```python
from build123d import *

# Parameters (mm, degrees)
SKETCH1_R               = 2.5
EXTRUDE_1_DEPTH         = 50
HOLE_WIZARD_5_5_5_5_1_D = 5.5
HOLE_WIZARD_5_5_5_5_2_D = 5.5


with BuildPart() as part:
    # Sketch1 → 凸台-拉伸1 (new body)
    with BuildSketch(Plane.XY):
        with BuildLine():
            Line((-6, -15), (-3.25, -15))
            Line((-3.25, -15), (-3.25, -13))
            Line((-3.25, -13), (-5, -13))
            Line((-5, -13), (-5, -6))
            Line((-5, -6), (-3.25, -6))
            Line((-3.25, -6), (-3.25, -4))
            Line((-3.25, -4), (3.25, -4))
            Line((3.25, -4), (3.25, -6))
            Line((3.25, -6), (5, -6))
            Line((5, -6), (5, -13))
            Line((5, -13), (3.25, -13))
            Line((3.25, -13), (3.25, -15))
            Line((3.25, -15), (6, -15))
            ThreePointArc((6, -15), (7.060660172, -14.560660172), (7.5, -13.5))
            Line((7.5, -13.5), (7.5, 13.5))
            ThreePointArc((7.5, 13.5), (7.060660172, 14.560660172), (6, 15))
            Line((6, 15), (3.25, 15))
            Line((3.25, 15), (3.25, 13))
            Line((3.25, 13), (5, 13))
            Line((5, 13), (5, 6))
            Line((5, 6), (3.25, 6))
            Line((3.25, 6), (3.25, 4))
            Line((3.25, 4), (-3.25, 4))
            Line((-3.25, 4), (-3.25, 6))
            Line((-3.25, 6), (-5, 6))
            Line((-5, 6), (-5, 13))
            Line((-5, 13), (-3.25, 13))
            Line((-3.25, 13), (-3.25, 15))
            Line((-3.25, 15), (-6, 15))
            ThreePointArc((-6, 15), (-7.060660172, 14.560660172), (-7.5, 13.5))
            Line((-7.5, 13.5), (-7.5, -13.5))
            ThreePointArc((-7.5, -13.5), (-7.060660172, -14.560660172), (-6, -15))
        make_face()
        Circle(SKETCH1_R, mode=Mode.SUBTRACT)
    extrude(amount=EXTRUDE_1_DEPTH)

    # Ø5.5 (5.5) 直径孔1 (through all)
    with Locations(Plane(origin=(7.5, 0, 0), x_dir=(0, 0, -1), z_dir=(1, 0, 0))):
        with Locations((-25, 0)):
            Hole(HOLE_WIZARD_5_5_5_5_1_D / 2)

    # Ø5.5 (5.5) 直径孔2 (through all)
    with Locations(Plane(origin=(7.5, 0, 0), x_dir=(0, 0, -1), z_dir=(1, 0, 0))):
        with Locations((-10, 0)):
            Hole(HOLE_WIZARD_5_5_5_5_2_D / 2)

    # 草图6 → M6 螺纹孔1 (revolve, cut)
    with BuildSketch(Plane(origin=(0, 0, 50), x_dir=(0, -1, 0), z_dir=(1, 0, 0))):
        Polygon((0, 0), (0, 26.502151548), (2.5, 25), (2.5, 0), align=None)
    revolve(axis=Axis((0, 0, 56.35), (0, 0, -1)), mode=Mode.SUBTRACT)


solid = part.part
```
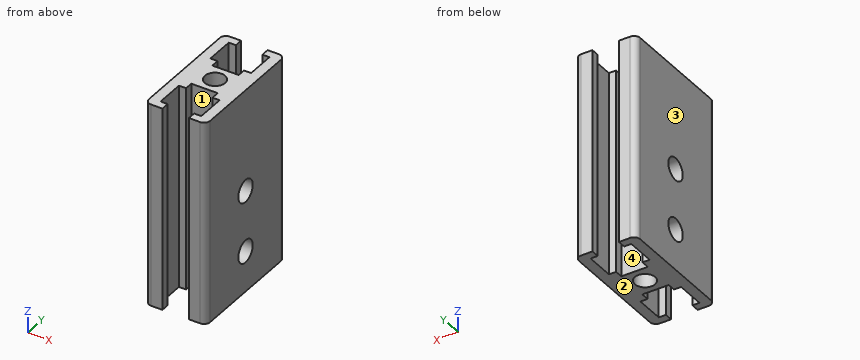
Geometry check sheet. Reference: the model listing, model coordinates, mm. Face numbers are marked on the shaded views. Coordinates: 2 decimals unless noted, no trailing zeros. Write each loop counter-clockwise with the first axis right and the second up, starting at its lowest first coordinate (ties: lowest second). Pieces come first, ordered by that corner, then holes. Notation, with made-up numbers: M 48,14.25 L 67,14.25 A23 ccw 67,43.25 Z; hole C -32.75,44 d9. An arc over 180 degrees is marked long. One line per item, written item: value. Start each with the question number.
(1) Release check for a two-part mould opening along X. For the marked faces 1, 2, 3 and 4 record: released by +X, released by -X, zero draft, split by the parting line, or undercut.
(2) Scan lines: line 1 along X through (y, z) = (0, 40.25); line 2 along Y through (x, z) = (-3.75, 25); line 3 along Y through (x, z) = (-3.75, 47.5). Record each from-to range of solid material in increasing order. Write a range as [from, to].
(3) Sectioned sample at C-C, the plane y = 0. Enter the section's corners in (x, z), and give its area (3 significant figures).
(4) Sectioned sample at A-A, the plane x = 0. Enter the section's corners in (y, z).
Filled sheet:
1. face 1: undercut
1. face 2: zero draft
1. face 3: released by -X
1. face 4: undercut
2. line 1: [-7.5, -2.5], [2.5, 7.5]
2. line 2: [-15, -13], [-6, -2.75], [2.75, 6], [13, 15]
2. line 3: [-15, -13], [-6, 6], [13, 15]
3. outline: M -7.5,0 L -2.5,0 L -2.5,7.25 L -7.5,7.25 Z; M -7.5,12.75 L -2.5,12.75 L -2.5,22.25 L -7.5,22.25 Z; M -7.5,27.75 L -2.5,27.75 L -2.5,50 L -7.5,50 Z; M 2.5,0 L 7.5,0 L 7.5,7.25 L 2.5,7.25 Z; M 2.5,12.75 L 7.5,12.75 L 7.5,22.25 L 2.5,22.25 Z; M 2.5,27.75 L 7.5,27.75 L 7.5,50 L 2.5,50 Z
3. area: 390 mm²
4. outline: M -4,0 L -2.5,0 L -2.5,8.85 A2.75 cw -2.5,11.15 L -2.5,23.85 A2.75 cw -2.5,26.15 L -2.5,50 L -4,50 Z; M 2.5,0 L 4,0 L 4,50 L 2.5,50 L 2.5,26.15 A2.75 cw 2.5,23.85 L 2.5,11.15 A2.75 cw 2.5,8.85 Z
